Verification items for the finished model (mm, model axes). A direction names the side the tool comes from. Coordinates: 2 decimals unless noted, no trailing zeros. Write each loop counter-clockwise with the first axis right and the second up, starting at its lowest first coordinate (ties: lowest second). Pieces come first, ordered by that corner, then holes. Notation, with made-up numbers: (34.5, -13.5) - (59.5, -13.5) arc R13 ccw to (59.5, 3.5) - close; hole circle Ø11 at (43.25, 70). An arc over 180 degrees is marked (long way). Use one line per item in the form item = value. Start each with the question number.
(1) Tool access check on faces 5 (the flat face through (7, -5.556, 1)), 6 (the flat face through (7, 3, 0)). Record the directions out of +Z, -Z, +X, -X, +Y, -Y that give a thin tool (end or side, any length) a straight path to the whole face; none if there is none.
(2) Sectioned sample at A-A (y = 1.5). Record the cut outline in (x, z).
(3) Sectioned sample at D-D (x = 5). Record the cut outline in (y, z).
(4) Gauge pin test, flat ends, axial feed: pin 1 Ø2 at (x, y) = (0, 9.13) entering from -Z; pin 2 Ø0.5 at (x, z) = (10, 0.5) entering from -Y. Record the tip position at first contact, or that the pin passes through.
(5) Material ranges on line 1 (Y direction, x = 0, z = 1.15); line 2 (Y direction, x = 16.5, z = 1.4); line 3 (X direction, y = 8.5, z = 0.55), recorded low to high. Write a range as [from, to].
(6) Sectioned sample at B-B (y = 10.5). Record the cut outline in (x, z), and give its area (3 significant figures).
(7) Mould release check, pull along X, two halves, no side actions. Record for faces 1 (the cylindrical face through (-0.387, 7.385, 0.783)), 2 (the cylindrical face through (18.1, 11.79, 0.8)), 3 (the cylindrical face through (15.531, 7.975, 0.783)), 4 (the cylindrical face through (-2.99, 11.08, 0.78)): released by +X, released by -X, zero draft, split by the parting line, or undercut.
(8) Sectioned sample at C-C (z = 1.25). Count the separate pieces of the cut face and the enclosed holes in it, and give its area (3 significant figures).
from build123d import *

# Parameters (mm, degrees)
SKETCH2_R           = 1.5875
SKETCH2_R_2         = 1.7859375
BOSS_EXTRUDE1_DEPTH = 1.5875
FILLET1_R           = 3.175
FILLET3_R           = 1.5875
FILLET2_R           = 0.508


with BuildPart() as part:
    # Sketch2 → Boss-Extrude1 (new body)
    with BuildSketch(Plane.XY):
        with BuildLine():
            ThreePointArc((-3.882150485, 3.975024739), (-5.145782024, -2.095910644), (0, -5.55625))
            Line((0, -5.55625), (14.2875, -5.55625))
            Line((14.2875, -5.55625), (14.2875, -7.18185))
            Line((14.2875, -7.18185), (17.4625, -7.18185))
            Line((17.4625, -7.18185), (17.4625, -5.55625))
            Line((17.4625, -5.55625), (19.05, -5.55625))
            Line((19.05, -5.55625), (19.05, 12.7))
            Line((19.05, 12.7), (0, 12.7))
            ThreePointArc((0, 12.7), (-3.017240848, 11.039812391), (-3.229688208, 7.602541474))
            ThreePointArc((-3.229688208, 7.602541474), (-2.975666516, 5.684416094), (-3.882150485, 3.975024739))
        make_face()
        with Locations((15.875, 9.525)):
            Circle(SKETCH2_R, mode=Mode.SUBTRACT)
        with Locations((15.875, -1.5875)):
            Circle(SKETCH2_R, mode=Mode.SUBTRACT)
        Circle(SKETCH2_R_2, mode=Mode.SUBTRACT)
        with Locations((0, 9.128125)):
            Circle(SKETCH2_R_2, mode=Mode.SUBTRACT)
    extrude(amount=BOSS_EXTRUDE1_DEPTH)

    # Fillet1
    fillet1_edges = [part.edges().sort_by_distance(p)[0] for p in [
        (19.05, 12.7, 0.79375),
    ]]
    fillet(fillet1_edges, radius=FILLET1_R)

    # Fillet3
    fillet3_edges = [part.edges().sort_by_distance(p)[0] for p in [
        (19.05, -5.55625, 0.79375),
    ]]
    fillet(fillet3_edges, radius=FILLET3_R - 0.0001)  # a hair under: the kernel refuses the full size

    # Fillet2
    fillet2_edges = [part.edges().sort_by_distance(p)[0] for p in [
        (17.4625, -5.55625, 0.79375),
        (17.4625, -7.18185, 0.79375),
        (14.2875, -7.18185, 0.79375),
        (14.2875, -5.55625, 0.79375),
    ]]
    fillet(fillet2_edges, radius=FILLET2_R)


solid = part.part
Answers below:
q1.face_5 = +Z, -Z, -X, -Y
q1.face_6 = -Z, +X, -X, +Y, -Y
q2.outline = (-5.35, 0) - (-0.97, 0) - (-0.97, 1.59) - (-5.35, 1.59) - close; (0.97, 0) - (19.05, 0) - (19.05, 1.59) - (0.97, 1.59) - close
q3.outline = (-5.56, 0) - (12.7, 0) - (12.7, 1.59) - (-5.56, 1.59) - close
q4.pin_1 = through
q4.pin_2 = -5.56
q5.line_1 = [-5.56, -1.79], [1.79, 7.34], [10.91, 12.7]
q5.line_2 = [-7.18, -3.05], [-0.13, 8.07], [10.98, 12.64]
q5.line_3 = [-3.52, -1.67], [1.67, 14.66], [17.09, 19.05]
q6.outline = (-3.3, 0) - (-1.14, 0) - (-1.14, 1.59) - (-3.3, 1.59) - close; (1.14, 0) - (14.62, 0) - (14.62, 1.59) - (1.14, 1.59) - close; (17.13, 0) - (18.9, 0) - (18.9, 1.59) - (17.13, 1.59) - close
q6.area = 27.6 mm2
q7.face_1 = undercut
q7.face_2 = released by +X
q7.face_3 = undercut
q7.face_4 = released by -X
q8.separate_pieces = 1
q8.enclosed_holes = 4
q8.area = 385 mm2
